```python
from build123d import *

# Parameters (mm, degrees)
F0_W          = 152.4
F0_H          = 2.54
F1_DEPTH      = 76.2
F1_DEPTH_BACK = 76.2
F2_W          = 116.0843670368
F2_H          = 27.2963345051
F3_DEPTH      = 25.4
F4_R          = 7.6032374963
F5_DEPTH      = 17.78
F6_R          = 3.3634669128
F7_T1_DEPTH   = 174.3970452561
F7_T3_DEPTH   = 174.3970452561


# Not quite as in the source:
# - a fillet or chamfer that OpenCascade refuses, or shapes differently, is made with other operations: its cross-section is extruded or revolved along the edge and cut away or added


with BuildPart() as f1:
    # F0 (on Front) → F1 (new body, two sides)
    with BuildSketch(Plane.XZ) as f1_sk:
        Rectangle(F0_W, F0_H)
    extrude(amount=-F1_DEPTH)
    extrude(f1_sk.sketch, amount=F1_DEPTH_BACK)

    # F2 (on face) → F3 (cut)
    with BuildSketch(Plane.XY.offset(1.27)):
        with Locations((0, 22.1970230341)):
            Rectangle(F2_W, F2_H)
    extrude(amount=-F3_DEPTH, mode=Mode.SUBTRACT)

    # F4 (on face) → F5 (join)
    with BuildSketch(Plane.XY.offset(1.27)):
        with Locations((0, -53.8427531719)):
            Circle(F4_R)
    extrude(amount=F5_DEPTH)

    # F6
    f6_edges = [f1.edges().sort_by_distance(p)[0] for p in [
        (7.603237, -53.842753, 10.16),
        (-7.603237, -53.842753, 1.27),
        (-7.603237, -53.842753, 19.05),
    ]]
    fillet(f6_edges, radius=F6_R)

    # F7: fillet of radius 5.08 on 4 edges, made by hand

    # F7_s2 → F7_t1 (cut)
    with BuildSketch(Plane.YZ.offset(-87.1985226281)):
        with BuildLine():
            ThreePointArc((-71.8005909488, 1.27), (-74.3405909488, 0.5894090512), (-76.2, -1.27))
            Line((-76.2, -1.27), (-76.2, 1.27))
            Line((-76.2, 1.27), (-71.8005909488, 1.27))
        make_face()
        with BuildLine():
            ThreePointArc((71.8005909488, 1.27), (74.3405909488, 0.5894090512), (76.2, -1.27))
            Line((76.2, -1.27), (76.2, 1.27))
            Line((76.2, 1.27), (71.8005909488, 1.27))
        make_face()
    extrude(amount=F7_T1_DEPTH, mode=Mode.SUBTRACT)

    # F7_s4 → F7_t3 (cut)
    with BuildSketch(Plane.XZ.offset(-87.1985226281)):
        with BuildLine():
            ThreePointArc((71.8005909488, 1.27), (74.3405909488, 0.5894090512), (76.2, -1.27))
            Line((76.2, -1.27), (76.2, 1.27))
            Line((76.2, 1.27), (71.8005909488, 1.27))
        make_face()
        with BuildLine():
            ThreePointArc((-71.8005909488, 1.27), (-74.3405909488, 0.5894090512), (-76.2, -1.27))
            Line((-76.2, -1.27), (-76.2, 1.27))
            Line((-76.2, 1.27), (-71.8005909488, 1.27))
        make_face()
    extrude(amount=F7_T3_DEPTH, mode=Mode.SUBTRACT)


solid = f1.part
```
Part model, mm, in its own coordinate system. A direction names the side the tool comes from. Coordinates: 2 decimals unless noted, no trailing zeros. Order: outer loops, then holes, each group sorted by start corner. A loop starts at its lowest first (then second) coordinate and runs counter-clockwise, first axis right, second up. Notation, with made-up numbers: (55, 63.25) -> (62, 63.25) arc R16 cw to (62, 90.25) -> close; hole circle Ø2 at (44, -29.5). An arc over 180 degrees is marked (long way). Put each result on its own line as item: value. Start each with the question number.
(1) Probe line 1 along Z through (x, y) = (4.5, 51.5); line 2 along X through (y, z) = (-58.5, 10.5). List the from-to ranges inside material, lowest first. Write a range as [from, to].
(2) Band-saw the part on C-C (x = 0). Give the cut face in (y, z).
(3) Band-saw the part on A-A (y = 13). Give the cut face in (x, z), then the cut area to 3 significant figures.
(4) Band-saw the part on B-B (x = -22). Give the cut face in (y, z), then the cut area to 3 significant figures.
(5) Pin check, flat tips, straight feed: pin 1 Ø2 at (y, z) = (23, -0.5) entering from +X; pin 2 Ø1.3 at (y, z) = (16, -0.5) entering from -X; pin 3 Ø2 at (x, z) = (-4, -0.5) entering from -Y. Stop position of each tip, or through.
(6) Band-saw the part on D-D (y = 46.5). Give the cut face in (x, z), then the cut area to 3 significant figures.
(7) Which spindle directions (+Z, -Z, +X, -X, +Y, -Y) get a long thin tool onto all of the face, cutting with end or side? Do faces 1 (the face through (-1, 1, -1.27)), 2 (the face through (-1.648, -61.265, 10.083)). Say none if no direction does.
Determined:
1. line 1: z = [-1.27, 1.27]
1. line 2: x = [-6.01, 6.01]
2. outline: (-76.2, -1.27) -> (8.55, -1.27) -> (8.55, 1.27) -> (-42.88, 1.27) arc R3.36 cw to (-46.24, 4.63) -> (-46.24, 15.69) arc R3.36 ccw to (-49.6, 19.05) -> (-58.08, 19.05) arc R3.36 ccw to (-61.45, 15.69) -> (-61.45, 4.63) arc R3.36 cw to (-64.81, 1.27) -> (-71.8, 1.27) arc R5.08 ccw to start; (35.85, -1.27) -> (76.2, -1.27) arc R5.08 ccw to (71.8, 1.27) -> (35.85, 1.27) -> close
3. outline: (-76.2, -1.27) -> (-58.04, -1.27) -> (-58.04, 1.27) -> (-71.8, 1.27) arc R5.08 ccw to start; (58.04, -1.27) -> (76.2, -1.27) arc R5.08 ccw to (71.8, 1.27) -> (58.04, 1.27) -> close
3. area: 85.7 mm²
4. outline: (-76.2, -1.27) -> (8.55, -1.27) -> (8.55, 1.27) -> (-71.8, 1.27) arc R5.08 ccw to start; (35.85, -1.27) -> (76.2, -1.27) arc R5.08 ccw to (71.8, 1.27) -> (35.85, 1.27) -> close
4. area: 311 mm²
5. pin 1: stops at x = 76.2
5. pin 2: stops at x = -76.13
5. pin 3: stops at y = -76.2
6. outline: (-76.2, -1.27) -> (76.2, -1.27) arc R5.08 ccw to (71.8, 1.27) -> (-71.8, 1.27) arc R5.08 ccw to start
6. area: 381 mm²
7. face 1: -Z, +X, -X, +Y, -Y
7. face 2: +Z
